from build123d import *

# Parameters (mm, degrees)
BOSS_EXTRUDE1_DEPTH = 5
BOSS_EXTRUDE2_DEPTH = 10
SKETCH3_R           = 1.5
SKETCH3_W           = 8
SKETCH3_H           = 8
SKETCH3_R_2         = 2.5
BOSS_EXTRUDE3_DEPTH = 7
SKETCH4_W           = 45
SKETCH4_H           = 10
SKETCH4_R           = 2.5
SKETCH4_W_2         = 1.788134659
SKETCH4_W_3         = 11.5
BOSS_EXTRUDE4_DEPTH = 7
FILLET1_R           = 3.5
SKETCH5_R           = 2.5
SKETCH5_R_2         = 2.55926668
SKETCH5_R_3         = 1.5
CUT_EXTRUDE1_DEPTH  = 123.977318254


with BuildPart() as part:
    # Sketch1 → Boss-Extrude1 (new body)
    with BuildSketch(Plane(origin=(0, 0, 0), x_dir=(1, 0, 0), z_dir=(0, 1, 0))):
        Polygon((-57.597316241, 51.805869074), (-57.597316241, -8.444130926), (-46.097316241, -28.194130926), (-46.097316241, -108.194130926), (43.902683759, -108.194130926), (43.902683759, -28.194130926), (55.402683759, -8.444130926), (55.402683759, 51.805869074), align=None)
    extrude(amount=BOSS_EXTRUDE1_DEPTH)

    # Sketch2 → Boss-Extrude2 (add)
    with BuildSketch(Plane(origin=(0, 5, 0), x_dir=(1, 0, 0), z_dir=(0, 1, 0))):
        Polygon((-46.097316241, -28.194130926), (-46.097316241, -108.194130926), (43.902683759, -108.194130926), (43.902683759, -28.194130926), (41.402683759, -28.194130926), (41.402683759, -105.694130926), (-43.597316241, -105.694130926), (-43.597316241, -28.194130926), align=None)
        Polygon((52.902683759, -6.988434723), (55.402683759, -8.444130926), (43.902683759, -28.194130926), (41.402683759, -26.738434723), align=None)
        Polygon((41.402683759, -28.194130926), (43.902683759, -28.194130926), (41.402683759, -26.738434723), align=None)
        Polygon((52.902683759, -6.988434723), (55.402683759, -8.444130926), (55.402683759, -6.988434723), align=None)
        Polygon((-57.597316241, 51.805869074), (-57.597316241, -6.988434723), (-55.097316241, -6.988434723), (-55.097316241, 49.305869074), (52.902683759, 49.305869074), (52.902683759, -6.988434723), (55.402683759, -6.988434723), (55.402683759, 51.805869074), align=None)
        Polygon((-43.597316241, -26.738434723), (-46.097316241, -28.194130926), (-43.597316241, -28.194130926), align=None)
        Polygon((-43.597316241, -26.738434723), (-46.097316241, -28.194130926), (-57.597316241, -8.444130926), (-55.097316241, -6.988434723), align=None)
        Polygon((-57.597316241, -6.988434723), (-57.597316241, -8.444130926), (-55.097316241, -6.988434723), align=None)
    extrude(amount=BOSS_EXTRUDE2_DEPTH)

    # Sketch3 → Boss-Extrude3 (add)
    # profile 1 of 3: a face of its own
    with BuildSketch(Plane(origin=(0, 5, 0), x_dir=(1, 0, 0), z_dir=(0, 1, 0))):
        Polygon((-43.597316241, -99.694130926), (-43.597316241, -105.694130926), (41.402683759, -105.694130926), (41.402683759, -99.694130926), (32.902683759, -99.694130926), (20.902683759, -102.694130926), (-23.097316241, -102.694130926), (-35.097316241, -99.694130926), align=None)
        with Locations(Location((-39.347316241, -101.944130926, 0), (0, 0, 270))):
            Circle(SKETCH3_R, mode=Mode.SUBTRACT)
        with Locations(Location((37.152683759, -101.944130926, 0), (0, 0, 270))):
            Circle(SKETCH3_R, mode=Mode.SUBTRACT)
    # profile 2 of 3: a face of its own
    with BuildSketch(Plane(origin=(0, 5, 0), x_dir=(1, 0, 0), z_dir=(0, 1, 0))):
        with Locations((-51.097316241, 45.305869074)):
            Rectangle(SKETCH3_W, SKETCH3_H)
        with Locations(Location((-51.097316241, 45.305869074, 0), (0, 0, 270))):
            Circle(SKETCH3_R_2, mode=Mode.SUBTRACT)
    # profile 3 of 3: a face of its own
    with BuildSketch(Plane(origin=(0, 5, 0), x_dir=(1, 0, 0), z_dir=(0, 1, 0))):
        with Locations((48.902683759, 45.305869074)):
            Rectangle(SKETCH3_W, SKETCH3_H)
        with Locations(Location((48.902683759, 45.305869074, 0), (0, 0, 270))):
            Circle(SKETCH3_R_2, mode=Mode.SUBTRACT)
    extrude(amount=BOSS_EXTRUDE3_DEPTH)

    # Sketch4 → Boss-Extrude4 (add)
    # profile 1 of 4: a face of its own
    with BuildSketch(Plane(origin=(0, 5, 0), x_dir=(1, 0, 0), z_dir=(0, 1, 0))):
        with Locations((-21.097316241, 5.130869074)):
            Rectangle(SKETCH4_W, SKETCH4_H)
        with Locations(Location((-31.847316241, 5.130869074, 0), (0, 0, 270))):
            Circle(SKETCH4_R, mode=Mode.SUBTRACT)
        with Locations(Location((-21.847316241, 5.130869074, 0), (0, 0, 270))):
            Circle(SKETCH4_R, mode=Mode.SUBTRACT)
    # profile 2 of 4: a face of its own
    with BuildSketch(Plane(origin=(0, 5, 0), x_dir=(1, 0, 0), z_dir=(0, 1, 0))):
        with Locations((40.50861643, 5.130869074)):
            Rectangle(SKETCH4_W_2, SKETCH4_H)
    # profile 3 of 4: a face of its own
    with BuildSketch(Plane(origin=(0, 5, 0), x_dir=(1, 0, 0), z_dir=(0, 1, 0))):
        with Locations((-49.347316241, 5.130869074)):
            Rectangle(SKETCH4_W_3, SKETCH4_H)
    # profile 4 of 4: a face of its own
    with BuildSketch(Plane(origin=(0, 5, 0), x_dir=(1, 0, 0), z_dir=(0, 1, 0))):
        with Locations((47.152683759, 5.130869074)):
            Rectangle(SKETCH4_W_3, SKETCH4_H)
    extrude(amount=BOSS_EXTRUDE4_DEPTH)

    # Fillet1
    fillet1_edges = [part.edges().sort_by_distance(p)[0] for p in [
        (41.402683759, 8.5, 99.694130926),
        (32.902683759, 8.5, 99.694130926),
        (20.902683759, 8.5, 102.694130926),
        (-23.097316241, 8.5, 102.694130926),
        (-35.097316241, 8.5, 99.694130926),
        (-43.597316241, 8.5, 99.694130926),
        (-47.097316241, 8.5, -41.305869074),
        (44.902683759, 8.5, -41.305869074),
        (55.402683759, 7.5, 8.444130926),
        (43.902683759, 7.5, 28.194130926),
        (43.902683759, 7.5, 108.194130926),
        (-46.097316241, 7.5, 108.194130926),
        (-46.097316241, 7.5, 28.194130926),
        (-57.597316241, 7.5, 8.444130926),
        (-57.597316241, 7.5, -51.805869074),
        (55.402683759, 7.5, -51.805869074),
        (52.902683759, 8.5, -10.130869074),
        (39.6145491, 8.5, -10.130869074),
        (39.6145491, 8.5, -0.130869074),
        (52.902683759, 8.5, -0.130869074),
        (1.402683759, 8.5, -10.130869074),
        (1.402683759, 8.5, -0.130869074),
        (-55.097316241, 8.5, -0.130869074),
        (-55.097316241, 8.5, -10.130869074),
        (-43.597316241, 10, 26.738434723),
        (-55.097316241, 10, 6.988434723),
        (52.902683759, 10, 6.988434723),
        (41.402683759, 10, 26.738434723),
    ]]
    fillet(fillet1_edges, radius=FILLET1_R)

    # Sketch5 → Cut-Extrude1 (cut, through all)
    with BuildSketch(Plane(origin=(0, 5, 0), x_dir=(1, 0, 0), z_dir=(0, 1, 0))):
        with Locations(Location((-21.847316241, 5.130869074, 0), (0, 0, 270))):
            Circle(SKETCH5_R)
        with Locations(Location((-31.847316241, 5.130869074, 0), (0, 0, 270))):
            Circle(SKETCH5_R_2)
        with Locations(Location((-39.347316241, -101.944130926, 0), (0, 0, 270))):
            Circle(SKETCH5_R_3)
        with Locations(Location((37.152683759, -101.944130926, 0), (0, 0, 270))):
            Circle(SKETCH5_R_3)
        with Locations(Location((-51.097316241, 45.305869074, 0), (0, 0, 270))):
            Circle(SKETCH5_R)
        with Locations(Location((48.902683759, 45.305869074, 0), (0, 0, 270))):
            Circle(SKETCH5_R)
    extrude(amount=-CUT_EXTRUDE1_DEPTH, mode=Mode.SUBTRACT)


solid = part.part
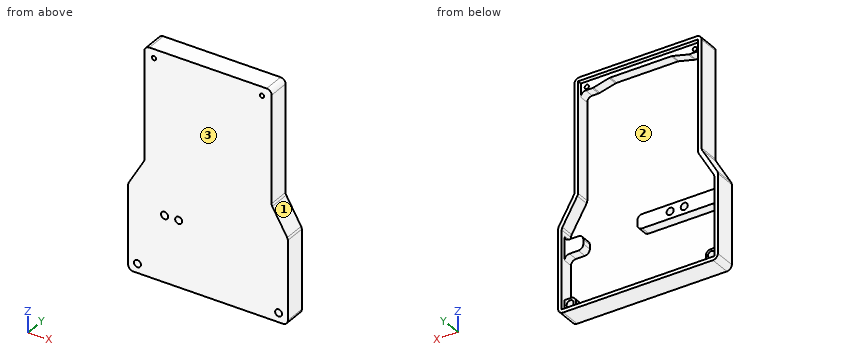
The model under review builds one solid part; all positions refer to its coordinate system, in mm. Face numbers are marked on the shaded views. Give positions to 0.01 mm unless a question says otherwise; leave off trailing zeros. Order: outer loops, then holes, each group sorted by start corner. A loop starts at its lowest first (then second) coordinate and runs counter-clockwise, first axis right, second up. Notation, with made-up numbers: (89, -9) -> (104, -9) arc R14 ccw to (104, 16) -> close; hole circle Ø11 at (-34.75, 53). An arc over 180 degrees is marked (long way). Write item = value, one per line. Start each with the question number.
(1) Take a section at C-C (y = 2.25). Write out the cut boundary in (x, z), plus the area to 3 significant figures.
(2) For L1, parallel to Z at x = -15.5, y = 11.5; L2, parallel to X at y = 12.25, z = 61; L3, parallel to Z at x = -36.5, y = 5.5, list the stretches that pass through material, from the lowest coordinate up. Write a range as from..to.
(3) Take a section at A-A (z = 79.5). Write out the cut boundary in (x, y), plus the area to 3 significant figures.
(4) Take a section at D-D (z = -15.5). Write out the cut boundary in (x, y).
(5) For pin 1 Ø5 at (x, z) = (-11, 102) entering from +Y; pin 2 Ø2 at (y, z) = (12, 68.5) entering from -X; pin 3 Ø5 at (y, z) = (10.5, 70.5) entering from +X; pin 4 Ø4 at (x, z) = (-21.85, -5.13) entering from +Y, all flat-tipped, find the tip position at first contact; note any pin that passes through.
(6) Take a section at B-B (x = -10). Write out the cut boundary in (y, z), plus the area to 3 significant figures.
(7) Draft analysis for pull direction Z (two halves, no side actions). For the marked faces 1, 2 and 3, state which applies: +Z half, -Z half, draft (parallel to the pull), parting line (faces both ways), or undercut.
Returned:
q1.outline = (-57.6, -48.31) arc R3.5 ccw to (-54.1, -51.81) -> (51.9, -51.81) arc R3.5 ccw to (55.4, -48.31) -> (55.4, 7.5) arc R3.5 ccw to (54.93, 9.26) -> (44.38, 27.38) arc R3.5 cw to (43.9, 29.14) -> (43.9, 104.69) arc R3.5 ccw to (40.4, 108.19) -> (-42.6, 108.19) arc R3.5 ccw to (-46.1, 104.69) -> (-46.1, 29.14) arc R3.5 cw to (-46.57, 27.38) -> (-57.12, 9.26) arc R3.5 ccw to (-57.6, 7.5) -> close; hole circle Ø5 at (-51.1, -45.31); hole circle Ø3 at (-39.35, 101.94); hole circle Ø5.12 at (-31.85, -5.13); hole circle Ø5 at (-21.85, -5.13); hole circle Ø3 at (37.15, 101.94); hole circle Ø5 at (48.9, -45.31)
q1.area = 15,900 mm²
q2.L1 = -51.81..-49.31, -10.13..-0.13, 102.69..108.19
q2.L2 = -46.1..-43.6, 41.4..43.9
q2.L3 = -51.81..-49.31, -10.13..-0.13, 99.69..108.19
q3.outline = (-46.1, 0) -> (43.9, 0) -> (43.9, 15) -> (41.4, 15) -> (41.4, 5) -> (-43.6, 5) -> (-43.6, 15) -> (-46.1, 15) -> close
q3.area = 500 mm²
q4.outline = (-57.6, 0) -> (55.4, 0) -> (55.4, 15) -> (52.9, 15) -> (52.9, 5) -> (-55.1, 5) -> (-55.1, 15) -> (-57.6, 15) -> close
q5.pin_1 = 12
q5.pin_2 = -46.1
q5.pin_3 = 43.9
q5.pin_4 = through
q6.outline = (0, -51.81) -> (15, -51.81) -> (15, -49.31) -> (5, -49.31) -> (5, -10.13) -> (12, -10.13) -> (12, -0.13) -> (5, -0.13) -> (5, 102.69) -> (12, 102.69) -> (12, 105.69) -> (15, 105.69) -> (15, 108.19) -> (0, 108.19) -> close
q6.area = 941 mm²
q7.face_1 = +Z half
q7.face_2 = undercut
q7.face_3 = draft
